from build123d import *

# Parameters (mm, degrees)
F0_W     = 100
F0_H     = 100
F1_DEPTH = 50
F2_W     = 102.432432
F2_H     = 50
F3_DEPTH = 50


with BuildPart() as f1:
    # F0 (on Top) → F1 (new body)
    with BuildSketch(Plane.XY):
        with Locations((4.56433, -14.662177)):
            Rectangle(F0_W, F0_H)
    extrude(amount=-F1_DEPTH)

    # F2 (on Top) → F3 (join)
    with BuildSketch(Plane.XY):
        with Locations((4.624579, 10.966863)):
            Rectangle(F2_W, F2_H)
    extrude(amount=F3_DEPTH)


solid = f1.part
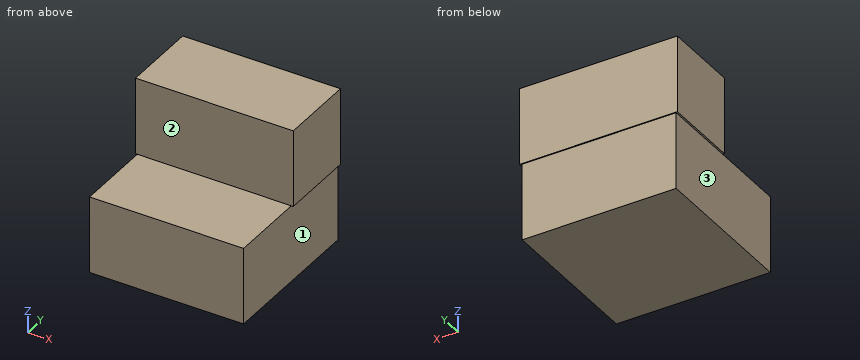
The model under review builds one solid part; all positions refer to its coordinate system, in mm. Face numbers are marked on the shaded views. A direction names the side the tool comes from. Round coordinates to 2 decimals unless told otherwise and drop trailing zeros. Write each loop counter-clockwise with the first axis right and the second up, starting at its lowest first coordinate (ties: lowest second). Pieces come first, ordered by that corner, then holes. Notation, with made-up numbers: (22.5, -39) -> (69.5, -39) arc R28 cw to (69.5, -20) -> close; hole circle Ø6 at (81, -28.5). An arc over 180 degrees is marked (long way). Answer as a JSON object with one key per item and string values.
1. We need section A-A on x = 47. State the section outline as (y, z) points.
Results found:
{"outline": "(-64.66, -50) -> (35.34, -50) -> (35.34, 0) -> (35.97, 0) -> (35.97, 50) -> (-14.03, 50) -> (-14.03, 0) -> (-64.66, 0) -> close"}
2. We need section C-C on y = -37.5. State the section outline as (x, z) points, and give its area (3 significant figures).
Results found:
{"outline": "(-45.44, -50) -> (54.56, -50) -> (54.56, 0) -> (-45.44, 0) -> close", "area": "5,000 mm^2"}
3. To check wall thickness, follow line 1 along X through (y, z) = (-55.5, -12); line 2 along Y through (x, z) = (-8, 6.5); line 3 along Z through (x, y) = (-5, -55). State the ranges of each line that lie inside material, in increasing order.
Results found:
{"line 1": "x = -45.44 to 54.56", "line 2": "y = -14.03 to 35.97", "line 3": "z = -50 to 0"}
4. Clearance check with flat-ended pins moving along their axes: pin 1 (15 mm diameter, centred on x = -19, y = -32, fed in from +Z); pin 2 (15 mm diameter, centred on x = -10.5, z = -15.5, fed in from +Y); pin 3 (4 mm diameter, centred on y = -5, z = -21, fed in from -X). State where each tip first meets the part, or that it passes through.
Results found:
{"pin 1": "stops at z = 0", "pin 2": "stops at y = 35.34", "pin 3": "stops at x = -45.44"}
5. We need section B-B on z = -17.5. State the section outline as (x, y) points.
Results found:
{"outline": "(-45.44, -64.66) -> (54.56, -64.66) -> (54.56, 35.34) -> (-45.44, 35.34) -> close"}
6. Machinability: for the marked faces 1, 2 and 3, which of the approach directions +Z, -Z, +X, -X, +Y, -Y give a long, thin tool a straight path to every point of the face, cutting with its end or side? Answer none if there is none.
Results found:
{"face 1": "-Z, +X, +Y, -Y", "face 2": "+Z, +X, -X, -Y", "face 3": "-Z, -X, +Y, -Y"}
